Verification items for the finished model (mm, model axes). Face numbers are marked on the shaded views. A direction names the side the tool comes from. Coordinates: 2 decimals unless noted, no trailing zeros. Order: outer loops, then holes, each group sorted by start corner. A loop starts at its lowest first (then second) coordinate and runs counter-clockwise, first axis right, second up. Notation, with made-up numbers: M 44.25,12 L 63.25,12 A23 cw 63.25,41 Z; hole C -0.75,20.5 d10. An arc over 180 degrees is marked long. Return JSON: item names as keys, results as strings. Group by question number.
1. Material ranges on line 1 along Y through (x, z) = (70.5, 17); line 2 along X through (y, z) = (37, 22.5), recorded low to high.
2. Mould release check, pull along X, two halves, no side actions. Record for the marked faces 1, 2 and 3: +X half, -X half, draft (parallel to the pull), parting line (faces both ways), or undercut.
3. Set-up check for the marked faces 4, 5 and 6: record each of +Z, -Z, +X, -X, +Y, -Y from which the full face is reachable in a straight line by a thin tool's end or side.
4. Section check B-B, the plane y = 27. Record the cut outline in (x, z), plus the area to 3 significant figures.
5. Gauge pin test, flat ends, axial feed: pin 1 (6.5 mm diameter, centred on y = 33.5, z = 16, fed in from -X); pin 2 (1.5 mm diameter, centred on y = 64.5, z = 15.5, fed in from +X). Record the tip position at first contact, or that the pin passes through.
6. Section check A-A, the plane z = 22. Record the cut outline in (x, y).
Autodesk Inventor part; units mm, degrees
ref_plane "YZ Plane" through (0, 0, 0) normal (1, 0, 0) x (0, 1, 0)
ref_plane "XZ Plane" through (0, 0, 0) normal (0, 1, 0) x (-1, 0, 0)
ref_plane "XY Plane" through (0, 0, 0) normal (0, 0, 1) x (1, 0, 0)
sketch "Sketch1" plane through (0, 0, 0) normal (0, 0, 1) x (1, 0, 0)
  line L0 (152.4, 12.7) -> (152.4, 76.2)
  line L1 (0, 76.2) -> (0, 0)
  line L2 (0, 76.2) -> (12.7, 76.2)
  line L3 (12.7, 76.2) -> (12.7, 63.5)
  line L4 (12.7, 63.5) -> (0, 63.5)
  line L5 (0, 63.5) -> (0, 76.2)
  line L6 (152.4, 76.2) -> (139.7, 76.2)
  line L7 (139.7, 76.2) -> (139.7, 63.5)
  line L8 (139.7, 63.5) -> (152.4, 63.5)
  line L9 (152.4, 63.5) -> (152.4, 76.2)
  line L10 (63.5, 76.2) -> (88.9, 76.2)
  line L11 (88.9, 76.2) -> (88.9, 63.5)
  line L12 (88.9, 63.5) -> (63.5, 63.5)
  line L13 (63.5, 63.5) -> (63.5, 76.2)
  line L14 (152.4, 76.2) -> (152.4, 88.9)
  line L15 (152.4, 88.9) -> (0, 88.9)
  line L16 (0, 88.9) -> (0, 76.2)
  line L17 (12.7, 38.1) -> (12.7, 25.4)
  line L18 (12.7, 25.4) -> (0, 25.4)
  line L19 (0, 25.4) -> (0, 38.1)
  line L20 (0, 38.1) -> (12.7, 38.1)
  line L21 (88.9, 25.4) -> (63.5, 25.4)
  line L22 (63.5, 25.4) -> (63.5, 38.1)
  line L23 (88.9, 38.1) -> (88.9, 25.4)
  line L24 (63.5, 38.1) -> (88.9, 38.1)
  line L25 (139.7, 38.1) -> (139.7, 25.4)
  line L26 (139.7, 25.4) -> (152.4, 25.4)
  line L27 (152.4, 25.4) -> (152.4, 38.1)
  line L28 (152.4, 38.1) -> (139.7, 38.1)
  line L29 (0, 76.2) -> (12.7, 76.2)
  line L30 (12.7, 76.2) -> (0, 76.2)
  line L31 (152.4, 76.2) -> (139.7, 76.2)
  line L32 (88.9, 76.2) -> (63.5, 76.2)
  line L33 (63.5, 76.2) -> (88.9, 76.2)
  line L34 (139.7, 76.2) -> (152.4, 76.2)
  line L35 (0, 12.7) -> (152.4, 12.7)
  point P0 (146.05, 76.2)
  point P1 (76.2, 76.2)
  point P2 (76.2, 38.1)
  point P3 (146.05, 38.1)
  point P4 (6.35, 25.4)
  point P5 (0, 63.5)
  point P6 (0, 25.4)
  dimension "d0" = 152.4
  dimension "d2" = 12.7
  dimension "d4" = 12.7
  dimension "d5" = 12.7
  dimension "d6" = 63.5
  dimension "d7" = 25.4
  dimension "d8" = 12.7
  dimension "d12" = 38.1
  dimension "d18" = 12.7
  dimension "d19" = 12.7
  dimension "d20" = 12.7
extrude "Extrusion1" add sketch "Sketch1" along normal blind 25.4 contours L35 L1 L18 L17 L20 L4 L3 L2 L16 L15 L14 L6 L7 L8 L0 L28 L25 L26
properties part number "Base"
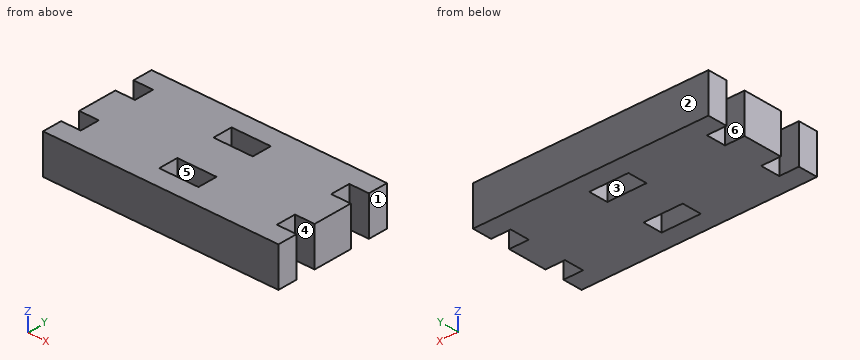
Answers follow:
{
 "1": {"line 1": "12.7 to 25.4, 38.1 to 63.5, 76.2 to 88.9", "line 2": "12.7 to 63.5, 88.9 to 139.7"},
 "2": {"face 1": "+X half", "face 2": "draft", "face 3": "undercut"},
 "3": {"face 4": "+Z, -Z, +X", "face 5": "+Z, -Z", "face 6": "+Z, -Z, -X"},
 "4": {"outline": "M 12.7,0 L 63.5,0 L 63.5,25.4 L 12.7,25.4 Z; M 88.9,0 L 139.7,0 L 139.7,25.4 L 88.9,25.4 Z", "area": "2,580 mm^2"},
 "5": {"pin 1": "x = 12.7", "pin 2": "x = 139.7"},
 "6": {"outline": "M 0,12.7 L 152.4,12.7 L 152.4,25.4 L 139.7,25.4 L 139.7,38.1 L 152.4,38.1 L 152.4,63.5 L 139.7,63.5 L 139.7,76.2 L 152.4,76.2 L 152.4,88.9 L 0,88.9 L 0,76.2 L 12.7,76.2 L 12.7,63.5 L 0,63.5 L 0,38.1 L 12.7,38.1 L 12.7,25.4 L 0,25.4 Z; hole M 63.5,25.4 L 88.9,25.4 L 88.9,38.1 L 63.5,38.1 Z; hole M 63.5,63.5 L 88.9,63.5 L 88.9,76.2 L 63.5,76.2 Z"}
}
